from build123d import *

# Parameters (mm, degrees)
F0_W     = 76.2
F0_H     = 76.2
F1_DEPTH = 38.1
F2_R     = 10.16
F3_DEPTH = 147.32
F4_R     = 10.16
F5_DEPTH = 163.322
F6_R     = 10.16
F7_DEPTH = 99.06
F8_R     = 5.08
F9_SIZE  = 2.54


with BuildPart() as f1:
    # F0 (on Top) → F1 (new body, symmetric)
    with BuildSketch(Plane.XY):
        Rectangle(F0_W, F0_H)
    extrude(amount=F1_DEPTH, both=True)

    # F2 (on face) → F3 (cut, symmetric)
    with BuildSketch(Plane(origin=(-38.1, 0, 0), x_dir=(0, -1, 0), z_dir=(-1, 0, 0))):
        Circle(F2_R)
    extrude(amount=F3_DEPTH, both=True, mode=Mode.SUBTRACT)

    # F4 (on face) → F5 (cut)
    with BuildSketch(Plane(origin=(0, 0, -38.1), x_dir=(1, 0, 0), z_dir=(0, 0, -1))):
        Circle(F4_R)
    extrude(amount=-F5_DEPTH, mode=Mode.SUBTRACT)

    # F6 (on face) → F7 (cut)
    with BuildSketch(Plane.XZ.offset(38.1)):
        Circle(F6_R)
    extrude(amount=-F7_DEPTH, mode=Mode.SUBTRACT)

    # F8
    f8_edges = [f1.edges().sort_by_distance(p)[0] for p in [
        (-38.1, 0, 38.1),
        (-38.1, -38.1, 0),
        (-38.1, 38.1, 0),
        (-38.1, 0, -38.1),
        (0, 38.1, -38.1),
        (0, -38.1, -38.1),
        (0, 38.1, 38.1),
        (0, -38.1, 38.1),
        (38.1, -38.1, 0),
        (38.1, 0, -38.1),
        (38.1, 38.1, 0),
        (38.1, 0, 38.1),
    ]]
    fillet(f8_edges, radius=F8_R)

    # F9
    f9_edges = [f1.edges().sort_by_distance(p)[0] for p in [
        (-10.16, 0, -38.1),
        (38.1, 10.16, 0),
        (-10.16, -38.1, 0),
        (-10.16, 38.1, 0),
        (-10.16, 0, 38.1),
        (-38.1, 10.16, 0),
    ]]
    chamfer(f9_edges, length=F9_SIZE)


solid = f1.part
Can you work these out from the model? Positions are in its coordinate system, mm. Give positions to 0.01 mm unless a question says otherwise; leave off trailing zeros. Loops run counter-clockwise (first coordinate to the right, second up) from the corner with the lowest first, then second, coordinate; pieces in that order, holes last. Notation, with made-up numbers: M -20,62 L -12,62 A8 ccw -12,73 Z; hole C 23,4 d3. An arc over 180 degrees is marked long. One line per item, written item: value.
1) Thinking about a two-plate mould opening in Z: for faces 1 (the face through (36.572, 36.651, -0.462)), 2 (the face through (-36.651, 0.462, -36.572)), 3 (the face through (-8.16, 6.257, 35.683)), 4 (the face through (35.72, 8.19, -6.28)), which applies, +Z half, -Z half, draft (parallel to the pull), parting line (faces both ways), or undercut?
Geometry check:
face 1: draft
face 2: -Z half
face 3: +Z half
face 4: undercut
2) Imagine slicing it at A-A on x = 0. Write out the boundary of the cut face in (y, z).
Geometry check:
outline: M -38.1,-33.02 A5.08 ccw -33.02,-38.1 L -12.7,-38.1 L -10.16,-35.56 L -10.16,-10.16 L -35.56,-10.16 L -38.1,-12.7 Z; M -38.1,12.7 L -35.56,10.16 L -10.16,10.16 L -10.16,35.56 L -12.7,38.1 L -33.02,38.1 A5.08 ccw -38.1,33.02 Z; M 10.16,-35.56 L 12.7,-38.1 L 33.02,-38.1 A5.08 ccw 38.1,-33.02 L 38.1,-12.7 L 35.56,-10.16 L 10.16,-10.16 Z; M 10.16,10.16 L 35.56,10.16 L 38.1,12.7 L 38.1,33.02 A5.08 ccw 33.02,38.1 L 12.7,38.1 L 10.16,35.56 Z
3) Please list where this line runs through material, in increasing order: line 1 (Z direction, x = -27.25, y = 0).
Geometry check:
line 1: z = -38.1 to -10.16, 10.16 to 38.1
4) I'm going to push a flat-ended pin straight in: pin 1 (3 mm diameter, centred on x = 0.5, y = 9.5, fed in from -Z). Where does the tip first touch, or does it pass through?
Geometry check:
pin 1: stops at z = -36.41
5) Imagine slicing it at C-C on y = -27.5. Write out the boundary of the cut face in (x, z).
Geometry check:
outline: M -38.1,-33.02 A5.08 ccw -33.02,-38.1 L 33.02,-38.1 A5.08 ccw 38.1,-33.02 L 38.1,33.02 A5.08 ccw 33.02,38.1 L -33.02,38.1 A5.08 ccw -38.1,33.02 Z; hole C 0,0 d20.32
